```python
from build123d import *

# Parameters (mm, degrees)
F1_DEPTH  = 9.55
F2_W      = 8.7
F2_H      = 1
F3_DEPTH  = 3
F4_SIZE   = 0.5
F6_DEPTH  = 5.65
F6_TAPER  = 5
F8_DEPTH  = 4
F8_TAPER  = 15
F9_W      = 12
F9_H      = 7
F10_DEPTH = 7
F11_R     = 3.5
F12_DEPTH = 10
F12_TAPER = 10
F13_R     = 2.5
F14_DEPTH = 4
F15_SIZE  = 1.25


with BuildPart() as f1:
    # F0 (on Front) → F1 (new body)
    with BuildSketch(Plane.XZ):
        with BuildLine():
            Line((50.5, 15.125), (-50.5, 15.125))
            ThreePointArc((-50.5, 15.125), (-51.9142135624, 14.5392135624), (-52.5, 13.125))
            Line((-52.5, 13.125), (-52.5, -13.125))
            ThreePointArc((-52.5, -13.125), (-51.9142135624, -14.5392135624), (-50.5, -15.125))
            Line((-50.5, -15.125), (50.5, -15.125))
            ThreePointArc((50.5, -15.125), (51.9142135624, -14.5392135624), (52.5, -13.125))
            Line((52.5, -13.125), (52.5, 13.125))
            ThreePointArc((52.5, 13.125), (51.9142135624, 14.5392135624), (50.5, 15.125))
        make_face()
    extrude(amount=F1_DEPTH)

    # F2 (on face) → F3 (join)
    with BuildSketch(Plane.XZ.offset(9.55)):
        with BuildLine():
            Line((44.5, 12.125), (-44.5, 12.125))
            ThreePointArc((-44.5, 12.125), (-48.0355339059, 10.6605339059), (-49.5, 7.125))
            Line((-49.5, 7.125), (-49.5, -7.125))
            ThreePointArc((-49.5, -7.125), (-48.0355339059, -10.6605339059), (-44.5, -12.125))
            Line((-44.5, -12.125), (44.5, -12.125))
            ThreePointArc((44.5, -12.125), (48.0355339059, -10.6605339059), (49.5, -7.125))
            Line((49.5, -7.125), (49.5, 7.125))
            ThreePointArc((49.5, 7.125), (48.0355339059, 10.6605339059), (44.5, 12.125))
        make_face()
        with Locations((-22, 0)):
            Rectangle(F2_W, F2_H, mode=Mode.SUBTRACT)
        with Locations((22, 0)):
            Rectangle(F2_W, F2_H, mode=Mode.SUBTRACT)
    extrude(amount=F3_DEPTH)

    # F4
    f4_edges = [f1.edges().sort_by_distance(p)[0] for p in [
        (-22, -12.55, 0.5),
        (-17.65, -12.55, 0),
        (-22, -12.55, -0.5),
        (-26.35, -12.55, 0),
        (22, -12.55, -0.5),
        (17.65, -12.55, 0),
        (22, -12.55, 0.5),
        (26.35, -12.55, 0),
    ]]
    chamfer(f4_edges, length=F4_SIZE)

    # F5 (on face) → F6 (join)
    with BuildSketch(Plane.XZ.offset(12.55)):
        with BuildLine():
            ThreePointArc((6.9988838396, -12.125), (12.1240334409, -7.000558058), (14, 0))
            ThreePointArc((14, 0), (12.1240334409, 7.000558058), (6.9988838396, 12.125))
            Line((6.9988838396, 12.125), (-6.9988838396, 12.125))
            ThreePointArc((-6.9988838396, 12.125), (-14, 0), (-6.9988838396, -12.125))
            Line((-6.9988838396, -12.125), (6.9988838396, -12.125))
        make_face()
        with BuildLine():
            Line((-6.9988838396, 12.125), (6.9988838396, 12.125))
            ThreePointArc((6.9988838396, 12.125), (0, 14), (-6.9988838396, 12.125))
        make_face()
        with BuildLine():
            ThreePointArc((-6.9988838396, -12.125), (0, -14), (6.9988838396, -12.125))
            Line((6.9988838396, -12.125), (-6.9988838396, -12.125))
        make_face()
    extrude(amount=F6_DEPTH, taper=F6_TAPER)

    # F7 (on face) → F8 (join)
    with BuildSketch(Plane(origin=(0, 0, 0), x_dir=(-1, 0, 0), z_dir=(0, 1, 0))):
        with BuildLine():
            ThreePointArc((49.5, 9), (48.6213203436, 11.1213203436), (46.5, 12))
            Line((46.5, 12), (-46.5, 12))
            ThreePointArc((-46.5, 12), (-48.6213203436, 11.1213203436), (-49.5, 9))
            Line((-49.5, 9), (-49.5, -9))
            ThreePointArc((-49.5, -9), (-48.6213203436, -11.1213203436), (-46.5, -12))
            Line((-46.5, -12), (46.5, -12))
            ThreePointArc((46.5, -12), (48.6213203436, -11.1213203436), (49.5, -9))
            Line((49.5, -9), (49.5, 9))
        make_face()
    extrude(amount=F8_DEPTH, taper=F8_TAPER)

    # F9 (on face) → F10 (join)
    with BuildSketch(Plane(origin=(0, 0, -15.125), x_dir=(1, 0, 0), z_dir=(0, 0, -1))):
        with Locations((0, 3.5)):
            Rectangle(F9_W, F9_H)
    extrude(amount=F10_DEPTH)

    # F11 (on face) → F12 (join)
    with BuildSketch(Plane(origin=(0, 4, 0), x_dir=(-1, 0, 0), z_dir=(0, 1, 0))):
        Circle(F11_R)
    extrude(amount=F12_DEPTH, taper=F12_TAPER)

    # F13 (on face) → F14 (join)
    with BuildSketch(Plane(origin=(0, 0, -22.125), x_dir=(1, 0, 0), z_dir=(0, 0, -1))):
        with Locations((0, 3.5)):
            Circle(F13_R)
    extrude(amount=F14_DEPTH)

    # F15
    f15_edges = [f1.edges().sort_by_distance(p)[0] for p in [
        (-2.5, -3.5, -26.125),
    ]]
    chamfer(f15_edges, length=F15_SIZE)


solid = f1.part
```
Verification items for the finished model (mm, model axes). A direction names the side the tool comes from. Give positions to 0.01 mm unless a question says otherwise; leave off trailing zeros. Order: outer loops, then holes, each group sorted by start corner. A loop starts at its lowest first (then second) coordinate and runs counter-clockwise, first axis right, second up. Notation, with made-up numbers: (87.5, 57) - (131.5, 57) arc R32 ccw to (131.5, 89) - close; hole circle Ø3 at (45.5, 69). An arc over 180 degrees is marked (long way). Answer as CSV lines item,"result". Start each with the question number.
Item 1: Mould release check, pull along Y, two halves, no side actions. Record for faces 1 (the face through (0, 14, 0)), 2 (the face through (0, -18.2, 0)), 3 (the face through (0, -12.55, 13)): released by +Y, released by -Y, zero draft, split by the parting line, or undercut.
Item 2: Gauge pin test, flat ends, axial feed: pin 1 (2 mm diameter, centred on y = -2.5, z = -19, fed in from +X); pin 2 (11 mm diameter, centred on x = -18, z = 0.5, fed in from +Y); pin 3 (12 mm diameter, centred on x = 36, z = 2, fed in from -Y). Record the tip position at first contact, or that the pin passes through.
Item 3: Access from +Z, -Z, +X, -X, +Y, -Y to the whole of each face (thin tool, end or side, straight path). Record for faces 4 (the face through (22, -11, -0.5)), 5 (the face through (6, -3, -19)), 6 (the face through (0, -7, -19)), 7 (the face through (-49.5, -11, 0)).
Item 4: Section check A-A, the plane y = -8.5. Record the boundary of the cut face in (x, z) (3 decimals).
Item 5: Section check B-B, the plane y = -3.5. Record the boundary of the cut face in (x, z) (3 decimals).
Item 6: Material ranges on L1, parallel to Z at x = -34, y = -4.5 (3 decimals); L2, parallel to Y at x = 27, z = 2; L3, parallel to Y at x = 26.5, z = 13, recorded low to high.
Filled in:
1,face 1,"released by +Y"
1,face 2,"released by -Y"
1,face 3,"undercut"
2,pin 1,"x = 6"
2,pin 2,"y = 4"
2,pin 3,"y = -12.55"
3,face 4,"-Y"
3,face 5,"-Z, +X, +Y, -Y"
3,face 6,"-Z, +X, -X, -Y"
3,face 7,"+Z, -Z, -X, -Y"
4,outline,"(-52.5, -13.125) arc R2 ccw to (-50.5, -15.125) - (50.5, -15.125) arc R2 ccw to (52.5, -13.125) - (52.5, 13.125) arc R2 ccw to (50.5, 15.125) - (-50.5, 15.125) arc R2 ccw to (-52.5, 13.125) - close"
5,outline,"(-52.5, -13.125) arc R2 ccw to (-50.5, -15.125) - (-6, -15.125) - (-6, -22.125) - (-2.5, -22.125) - (-2.5, -24.875) - (-1.25, -26.125) - (1.25, -26.125) - (2.5, -24.875) - (2.5, -22.125) - (6, -22.125) - (6, -15.125) - (50.5, -15.125) arc R2 ccw to (52.5, -13.125) - (52.5, 13.125) arc R2 ccw to (50.5, 15.125) - (-50.5, 15.125) arc R2 ccw to (-52.5, 13.125) - close"
6,L1,"-15.125 to 15.125"
6,L2,"-12.55 to 4"
6,L3,"-9.55 to 0"
